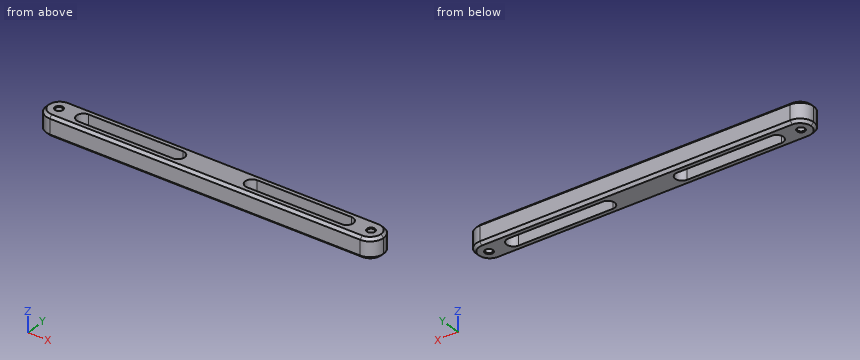
Autodesk Inventor part; units mm, degrees
ref_plane "YZ Plane" through (0, 0, 0) normal (1, 0, 0) x (0, 1, 0)
ref_plane "XZ Plane" through (0, 0, 0) normal (0, 1, 0) x (-1, 0, 0)
ref_plane "XY Plane" through (0, 0, 0) normal (0, 0, 1) x (1, 0, 0)
sketch "Skizze1" plane through (0, 0, 0) normal (0, 0, 1) x (1, 0, 0)
  line L0 (-175, 0) -> (175, 0) construction
  line L1 (0, 14) -> (0, -14) construction
  line L2 (-125, -10) -> (125, -10)
  line L3 (125, -10) -> (125, 10)
  line L4 (125, 10) -> (-125, 10)
  line L5 (-125, 10) -> (-125, -10)
  line L6 (-125, -10) -> (125, 10) construction
  line L7 (125, -10) -> (-125, 10) construction
  point P0 (0, 0)
  dimension "d0" = 250
  dimension "d1" = 20
extrude "Grundkörper" add sketch "Skizze1" along normal mid plane 15
sketch "Skizze2" plane through (0, 0, 7.5) normal (0, 0, 1) x (1, 0, 0)
  line L0 (0, 14) -> (0, -14) construction
  point P0 (0, 0)
  point P1 (-115.6, 0)
  point P2 (115.6, 0)
  dimension "d4" = 231.2
hole "M6" at (-115.6, 0, 7.5) at (115.6, 0, 7.5) direction (0, 0, -1) diameter 4.917 end through all
sketch "Skizze3" plane through (0, 0, 7.5) normal (0, 0, 1) x (1, 0, 0)
  line L0 (0, 14) -> (0, -14) construction
  line L1 (-97.5, 5) -> (-27.5, 5)
  line L2 (-22.5, 0) -> (-22.5, 0)
  line L3 (-27.5, -5) -> (-97.5, -5)
  line L4 (-102.5, 0) -> (-102.5, 0)
  line L5 (-212.2426, 0) -> (181.2071, 0) construction
  line L6 (125, 10) -> (-125, 10)
  line L7 (0, 10) -> (-125, 10)
  line L8 (-62.5, 10) -> (-62.5, -10) construction
  line L9 (-125, -10) -> (125, -10) construction
  arc A0 (-102.5, 0) -> (-97.5, -5) centre (-97.5, 0) ccw
  arc A1 (-97.5, 5) -> (-102.5, 0) centre (-97.5, 0) ccw
  arc A2 (-22.5, 0) -> (-27.5, 5) centre (-27.5, 0) ccw
  arc A3 (-27.5, -5) -> (-22.5, 0) centre (-27.5, 0) ccw
  point P0 (0, 0)
  point P1 (-102.5, 5)
  point P2 (-22.5, 5)
  dimension "d16" = 10
  dimension "d17" = 80
  dimension "d18" = 5
extrude "Ausschnitt_Gewichtsreduktion" cut sketch "Skizze3" against normal through all
mirror "Spiegeln_Ausschnitt_Gewichtsreduktion" about plane through (0, 0, 0) normal (1, 0, 0) of "Ausschnitt_Gewichtsreduktion"
chamfer "Fase_M6_Gewinde" distance 0.5 angle 45 4 edges at (-115.6, 2.4585, -7.5) (-115.6, 2.4585, 7.5) (115.6, 2.4585, 7.5) (115.6, 2.4585, -7.5)
fillet "Abrundung" radius 10 4 edges at (-125, 10, 0) (-125, -10, 0) (125, -10, 0) (125, 10, 0)
chamfer "Fase2" distance 2 angle 45 8 edges at (0, -10, 7.5) (122.0711, -7.0711, 7.5) (0, 10, 7.5) (-122.0711, 7.0711, 7.5) (0, -10, -7.5) (-122.0711, 7.0711, -7.5) (0, 10, -7.5) (122.0711, -7.0711, -7.5)
properties part number "200-60-DIFFERENTIAL-BAR-03" material "Aluminium 6061"
Can you work these out from the model? Positions are in its coordinate system, mm. Coordinates: 2 decimals unless noted, no trailing zeros. Order: outer loops, then holes, each group sorted by start corner. A loop starts at its lowest first (then second) coordinate and runs counter-clockwise, first axis right, second up. Notation, with made-up numbers: M 57.5,-10.5 L 84.5,-10.5 A22 ccw 84.5,-2.5 Z; hole C 57,89 d1. An arc over 180 degrees is marked long. Answer as CSV lines item,"result".
(1) I'm going to push flat-ended pins straight in: pin 1 (1.5 mm diameter, centred on y = 7, z = 5.5, fed in from -X); pin 2 (2 mm diameter, centred on x = 71.5, y = -3.5, fed in from -Z); pin 3 (6.5 mm diameter, centred on x = 115.6, y = 0, fed in from -Z); pin 4 (4 mm diameter, centred on y = -7, z = -1.5, fed in from -X). Where does each tip first touch, or does it pass through?
Geometry check:
pin 1,"x = -122.81"
pin 2,"through"
pin 3,"z = -7.5"
pin 4,"x = -123.66"
(2) Suppose I cut it at C-C on x = 106. Please give me the cut outline in (y, z), plus the area to 3 significant figures.
Geometry check:
outline,"M -10,-5.5 L -8,-7.5 L 8,-7.5 L 10,-5.5 L 10,5.5 L 8,7.5 L -8,7.5 L -10,5.5 Z"
area,"292 mm^2"
(3) Suppose I cut it at A-A on z = 0.25. Count the separate pieces of the cut face and the enclosed holes in it, plus the area to 3 significant figures.
Geometry check:
separate pieces,"1"
enclosed holes,"4"
area,"3,320 mm^2"
(4) Please list where these lines run through material, in increasing order: L1, parallel to X at y = 0, z = 0; L2, parallel to Y at x = -115.6, z = -2; L3, parallel to Y at x = 48, z = -2.
Geometry check:
L1,"-125 to -118.06, -113.14 to -102.5, -22.5 to 22.5, 102.5 to 113.14, 118.06 to 125"
L2,"-9.98 to -2.46, 2.46 to 9.98"
L3,"-10 to -5, 5 to 10"
(5) Suppose I cut it at B-B on x = -67.5. Please give me the cut outline in (y, z), plus the area to 3 significant figures.
Geometry check:
outline,"M -10,-5.5 L -8,-7.5 L -5,-7.5 L -5,7.5 L -8,7.5 L -10,5.5 Z; M 5,-7.5 L 8,-7.5 L 10,-5.5 L 10,5.5 L 8,7.5 L 5,7.5 Z"
area,"142 mm^2"
